Could you check a few things on this model? Use its own coordinates, in mm. A direction names the side the tool comes from. Coordinates: 2 decimals unless noted, no trailing zeros. Order: outer loops, then holes, each group sorted by start corner. A loop starts at its lowest first (then second) coordinate and runs counter-clockwise, first axis right, second up. Notation, with made-up numbers: (12.25, -26) - (37.25, -26) arc R23 cw to (37.25, -18) - close; hole circle Ø1 at (28, 84). An arc over 180 degrees is marked (long way). Answer as CSV lines item,"result". Start each with the question number.
1. I want a section at A-A, the plane x = 0. List the corners of the cut face in (y, z) for me.
2. Thinking about a two-plate mould opening in X: for faces 3 (the face through (-3.05, -13.72, 32.19)), 4 (the face through (36.8, 11.6, 9.4)), 5 (the face through (17, 1, 0)), which applies, released by +X, released by -X, zero draft, split by the parting line, or undercut?
3. I want a section at C-C, the plane z = 44. List the corners of the cut face in (x, y) for me, and give its area (3 significant figures).
4. I want a section at D-D, the plane x = 33. List the corners of the cut face in (y, z) for me.
5. I need wall thicknesses on probe 1 along Y at (x, z) = (0, 39); probe 2 along Y at (x, z) = (0, 14); probe 3 along X at (y, z) = (6.5, 22). Which ranges of each line are inside material? Lowest first, please.
6. For pin 1 (5 mm diameter, centred on y = 0.5, z = 31.5, fed in from +X); pin 2 (8 mm diameter, centred on x = 17, z = 12.5, fed in from +Y); pin 3 (2 mm diameter, centred on x = -22.5, z = 52.5, fed in from +Y); pin 4 (6 mm diameter, centred on y = -21.5, z = 56.5, fed in from +X), each with a flat end and sliding along its axis, tell me the tip position at first contact or that it passes through.
7. For faces 1 (the face through (20.38, 6.42, 40.96)), 2 (the face through (4, -14, 63.5)), which set-ups out of +Z, -Z, +X, -X, +Y, -Y let a thin tool reach every point of the face, with its end or its side?
from build123d import *

# Parameters (mm, degrees)
F0_R     = 38.583475
F1_DEPTH = 19.05
F2_R     = 21.368169
F3_DEPTH = 44.45
F4_R     = 14.054868
F5_DEPTH = 63.5
F6_DEPTH = 63.5


with BuildPart() as f1:
    # F0 (on Top) → F1 (new body)
    with BuildSketch(Plane.XY):
        Circle(F0_R)
    extrude(amount=F1_DEPTH)

    # F2 (on face) → F3 (join)
    with BuildSketch(Plane.XY.offset(19.05)):
        Circle(F2_R)
    extrude(amount=F3_DEPTH)

    # F4 (on face) → F5 (join)
    with BuildSketch(Plane.XY.offset(63.5)):
        Circle(F4_R)
    extrude(amount=-F5_DEPTH)

    # F4 (on face) → F6 (cut)
    with BuildSketch(Plane.XY.offset(63.5)):
        Circle(F4_R)
    extrude(amount=-F6_DEPTH, mode=Mode.SUBTRACT)


solid = f1.part
Solved:
1,outline,"(-38.58, 0) - (-14.05, 0) - (-14.05, 63.5) - (-21.37, 63.5) - (-21.37, 19.05) - (-38.58, 19.05) - close; (14.05, 0) - (38.58, 0) - (38.58, 19.05) - (21.37, 19.05) - (21.37, 63.5) - (14.05, 63.5) - close"
2,face 3,"undercut"
2,face 4,"split by the parting line"
2,face 5,"zero draft"
3,outline,"circle Ø42.74 at (0, 0); hole circle Ø28.11 at (0, 0)"
3,area,"814 mm2"
4,outline,"(-19.99, 0) - (19.99, 0) - (19.99, 19.05) - (-19.99, 19.05) - close"
5,probe 1,"y = -21.37 to -14.05, 14.05 to 21.37"
5,probe 2,"y = -38.58 to -14.05, 14.05 to 38.58"
5,probe 3,"x = -20.36 to -12.46, 12.46 to 20.36"
6,pin 1,"stops at x = 21.37"
6,pin 2,"stops at y = 36.33"
6,pin 3,"passes through"
6,pin 4,"stops at x = 10.69"
7,face 1,"+Z"
7,face 2,"+Z, +X, -X, +Y, -Y"
